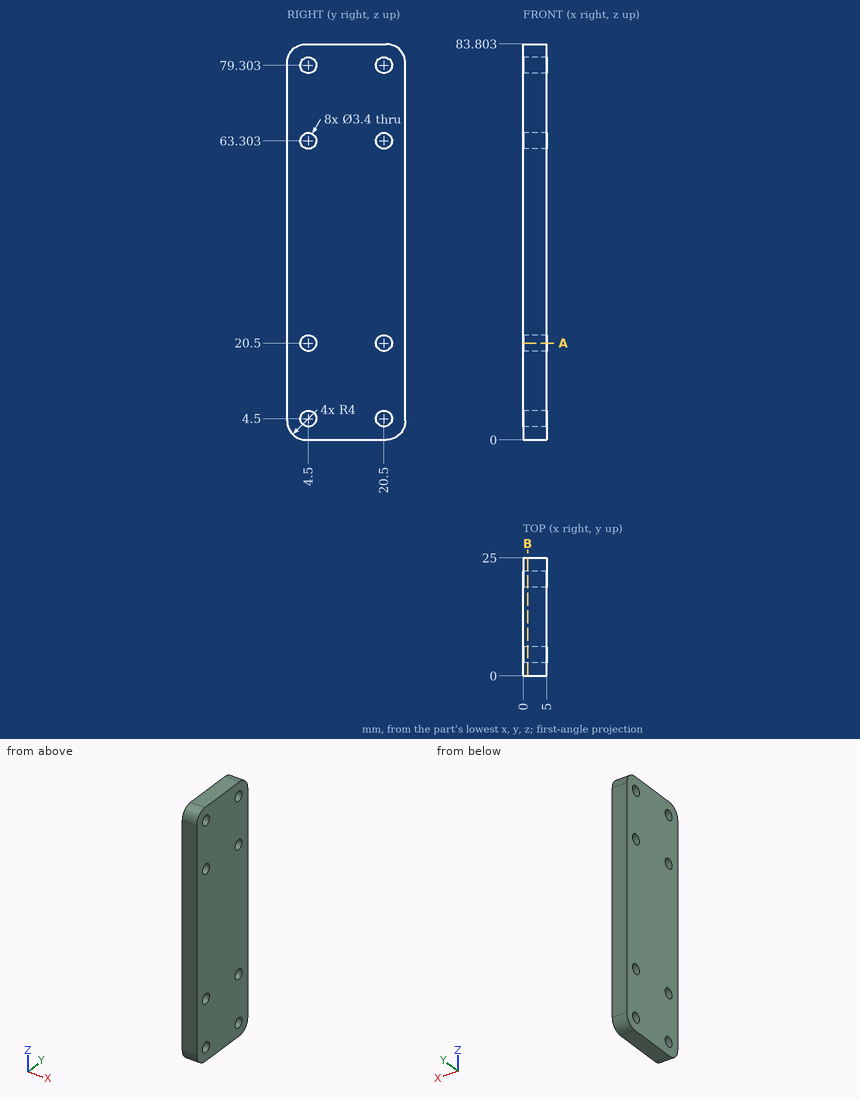
The drawing under review shows one solid part. Ordinate dimensions are in mm from its lowest x, y, z. Coordinates: 2 decimals unless noted, no trailing zeros. Write each loop counter-clockwise with the first axis right and the second up, starting at its lowest first coordinate (ties: lowest second). Pieces come first, ordered by that corner, then holes. Notation, with made-up numbers: M 78,-12 L 127,-12 A13 ccw 127,8 Z; hole C -18.75,16 d4. An arc over 180 degrees is marked long. Put each result on its own line as item: value.
1) Wall thickness on probe 1 along Y at (x, z) = (2.5, 20.5); probe 2 along Z at (x, y) = (3.25, 5) (1 decimal); probe 3 along Y at (x, z) = (0.7, 19.5) (1 decimal): over which ranges is each line inside the solid? List them lowest first. Write a range as [from, to].
Computed:
probe 1: y = [0, 2.8], [6.2, 18.8], [22.2, 25]
probe 2: z = [0, 2.9], [6.1, 18.9], [22.1, 61.7], [64.9, 77.7], [80.9, 83.8]
probe 3: y = [0, 3.1], [5.9, 19.1], [21.9, 25]
2) Clearance check with a flat-ended pin moving along its axis: pin 1 Ø3 at (y, z) = (4.5, 63.3) entering from -X. State where the tip first meets the part, or that it passes through.
Computed:
pin 1: passes through
3) Add section B-B on x = 0.95. State how many separate pieces and enclosed holes the cut face has, then the cut area to 3 significant figures.
Computed:
separate pieces: 1
enclosed holes: 8
area: 2,010 mm2
4) Add section A-A on z = 20.5. Give the boundary of the cut face in (x, y).
Computed:
outline: M 0,0 L 5,0 L 5,2.8 L 0,2.8 Z; M 0,6.2 L 5,6.2 L 5,18.8 L 0,18.8 Z; M 0,22.2 L 5,22.2 L 5,25 L 0,25 Z
